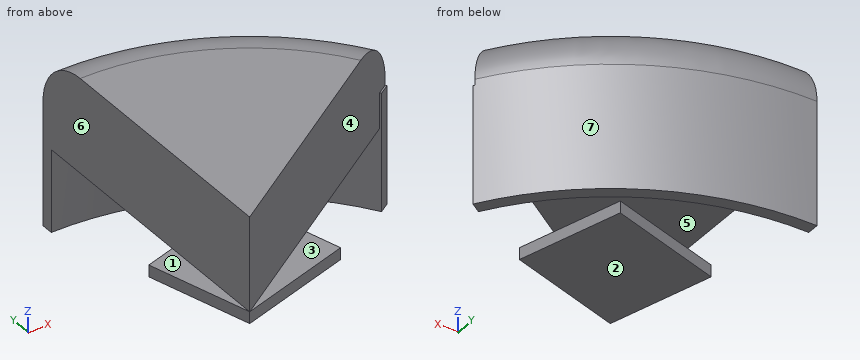
from build123d import *

# Parameters (mm, degrees)
BOX002_W               = 10
BOX002_H               = 9
BOX002_DEPTH           = 1
BOX002_PLACEMENT_ANGLE = 16
CYLINDER001_R          = 22
CYLINDER001_DEPTH      = 37
CYLINDER_R             = 25
CYLINDER_DEPTH         = 40
CYLINDER004_R          = 21
CYLINDER004_DEPTH      = 21
CYLINDER003_R          = 23
CYLINDER003_DEPTH      = 10
CYLINDER002_R          = 25
CYLINDER002_DEPTH      = 5
FILLET_R               = 4.5
BOX001_W               = 37
BOX001_H               = 39
BOX001_DEPTH           = 10
BOX001_PLACEMENT_ANGLE = 57
BOX_W                  = 37
BOX_H                  = 39
BOX_DEPTH              = 10
BOX004_W               = 33
BOX004_H               = 70
BOX004_DEPTH           = 17
BOX003_W               = 33
BOX003_H               = 70
BOX003_DEPTH           = 17
BOX003_PLACEMENT_ANGLE = 57
CYLINDER006_R          = 24
CYLINDER006_DEPTH      = 10
CYLINDER005_R          = 25
CYLINDER005_DEPTH      = 10


with BuildPart() as cubo002:
    # Box002 → Box002 (new body)
    with BuildSketch(Plane.XY):
        with Locations((5, 4.5)):
            Rectangle(BOX002_W, BOX002_H)
    extrude(amount=BOX002_DEPTH)


with BuildPart() as cubo002_1:
    # Box002 placement: moved
    add(cubo002.part.moved(Location((0, 0, 36))).rotate(Axis((0, 0, 36), (0, 0, 1)), BOX002_PLACEMENT_ANGLE))


with BuildPart() as cilindro001:
    # Cylinder001 → Cylinder001 (new body)
    with BuildSketch(Plane.XY):
        Circle(CYLINDER001_R)
    extrude(amount=CYLINDER001_DEPTH)


with BuildPart() as cut:
    # Cylinder → Cylinder (new body)
    with BuildSketch(Plane.XY):
        Circle(CYLINDER_R)
    extrude(amount=CYLINDER_DEPTH)

    # Cut: cut Cilindro001
    add(cilindro001.part, mode=Mode.SUBTRACT)


with BuildPart() as cilindro004:
    # Cylinder004 → Cylinder004 (new body)
    with BuildSketch(Plane.XY):
        Circle(CYLINDER004_R)
    extrude(amount=CYLINDER004_DEPTH)


with BuildPart() as cut001:
    # Cylinder003 → Cylinder003 (new body)
    with BuildSketch(Plane.XY):
        Circle(CYLINDER003_R)
    extrude(amount=CYLINDER003_DEPTH)

    # Cut001: cut Cilindro004
    add(cilindro004.part, mode=Mode.SUBTRACT)


with BuildPart() as cut001_1:
    # Cut001 placement: moved
    add(cut001.part.moved(Location((0, 0, -5))))


with BuildPart() as fusion:
    # Cylinder002 → Cylinder002 (new body)
    with BuildSketch(Plane.XY.offset(40)):
        Circle(CYLINDER002_R)
    extrude(amount=CYLINDER002_DEPTH)

    # Fillet
    fillet_edges = [fusion.edges().sort_by_distance(p)[0] for p in [
        (-25, 0, 45),
    ]]
    fillet(fillet_edges, radius=FILLET_R)

    # Fusion: union Cut, Cut001
    add(cut.part)
    add(cut001_1.part)


with BuildPart() as cubo001:
    # Box001 → Box001 (new body)
    with BuildSketch(Plane.XY):
        with Locations((18.5, 19.5)):
            Rectangle(BOX001_W, BOX001_H)
    extrude(amount=BOX001_DEPTH)


with BuildPart() as cubo001_1:
    # Box001 placement: moved
    add(cubo001.part.moved(Location((0, 0, 37))).rotate(Axis((0, 0, 37), (0, 0, -1)), BOX001_PLACEMENT_ANGLE))


with BuildPart() as common:
    # Box → Box (new body)
    with BuildSketch(Plane.XY.offset(37)):
        with Locations((18.5, 19.5)):
            Rectangle(BOX_W, BOX_H)
    extrude(amount=BOX_DEPTH)

    # Cut002: cut Cubo001
    add(cubo001_1.part, mode=Mode.SUBTRACT)

    # Common: intersect Fusion
    add(fusion.part, mode=Mode.INTERSECT)


with BuildPart() as cubo004:
    # Box004 → Box004 (new body)
    with BuildSketch(Plane(origin=(-33, -19, 29), x_dir=(1, 0, 0), z_dir=(0, 0, 1))):
        with Locations((16.5, 35)):
            Rectangle(BOX004_W, BOX004_H)
    extrude(amount=BOX004_DEPTH)


with BuildPart() as fusion001:
    # Box003 → Box003 (new body)
    with BuildSketch(Plane.XY):
        with Locations((16.5, 35)):
            Rectangle(BOX003_W, BOX003_H)
    extrude(amount=BOX003_DEPTH)


with BuildPart() as fusion001_1:
    # Box003 placement: moved
    add(fusion001.part.moved(Location((-29, -19, 29))).rotate(Axis((-29, -19, 29), (0, 0, -1)), BOX003_PLACEMENT_ANGLE))

    # Fusion001: union Cubo004
    add(cubo004.part)


with BuildPart() as cilindro006:
    # Cylinder006 → Cylinder006 (new body)
    with BuildSketch(Plane.XY.offset(34)):
        Circle(CYLINDER006_R)
    extrude(amount=CYLINDER006_DEPTH)


with BuildPart() as fusion002:
    # Cylinder005 → Cylinder005 (new body)
    with BuildSketch(Plane.XY.offset(34)):
        Circle(CYLINDER005_R)
    extrude(amount=CYLINDER005_DEPTH)

    # Cut003: cut Cilindro006
    add(cilindro006.part, mode=Mode.SUBTRACT)

    # Cut004: cut Fusion001
    add(fusion001_1.part, mode=Mode.SUBTRACT)


with BuildPart() as fusion002_1:
    # Cut004 placement: moved
    add(fusion002.part.moved(Location((0, 0, -4))))

    # Fusion002: union Cubo002, Common
    add(cubo002_1.part)
    add(common.part)


solid = fusion002_1.part
Source: CAD feature listing. Evaluate the final solid. Frame: model axes, mm. Face numbers are marked on the shaded views. A direction names the side the tool comes from. Round coordinates to 2 decimals unless told otherwise and drop trailing zeros. Loops run counter-clockwise (first coordinate to the right, second up) from the corner with the lowest first, then second, coordinate; pieces in that order, holes last. Notation, with made-up numbers: M 23,-28.75 L 57,-28.75 A19 cw 57,-5.75 Z; hole C 52,-27.75 d7. An arc over 180 degrees is marked long. Return JSON: item names as keys, results as strings. Group by question number.
1. Mould query, pull axis Y, two halves, no side actions, for the marked faces 4, 5, 6 and 7. Classes: released by +Y, released by -Y, zero draft, split by the parting line, or undercut.
2. Pin query (flat end, axial travel): pin 1 (0.7 mm diameter, centred on x = 20.5, y = 13.5, fed in from +Z); pin 2 (1 mm diameter, centred on x = 12.5, y = 14, fed in from -Z); pin 3 (8 mm diameter, centred on x = 14, z = 32, fed in from +Y); pin 4 (1.5 mm diameter, centred on y = 7.5, z = 35, fed in from +X). Return the tip coordinate at first contact, or that it passes through.
3. Reachability of the marked faces 1, 2 and 3 from +Z, -Z, +X, -X, +Y, -Y: full face, straight path, thin tool, end or side. Return the list, or none.
4. Section query A-A on y = 4.75. Output: boundary loops of the cut face in (x, z).
5. Material intervals for line 1 along Z through (x, y) = (4.25, 8.5); line 2 along Z through (x, y) = (-0.5, 3); line 3 along X through (y, z) = (14, 34.75), sorted ascending. Write a range as from..to.
6. Section query D-D on z = 41.5. Output: boundary loops of the cut face in (x, y).
7. Section query C-C on z = 38.25. Output: boundary loops of the cut face in (x, y).
8. Section query B-B on z = 35.5. Output: boundary loops of the cut face in (x, y).
Checks:
{
 "1": {"face 4": "released by -Y", "face 5": "undercut", "face 6": "zero draft", "face 7": "released by +Y"},
 "2": {"pin 1": "stops at z = 43.07", "pin 2": "stops at z = 37", "pin 3": "stops at y = 22.91", "pin 4": "passes through"},
 "3": {"face 1": "+Z, -X, +Y, -Y", "face 2": "-Z, +X, -X, -Y", "face 3": "+Z, +X, -Y"},
 "4": {"outline": "M -1.36,36 L 9.04,36 L 9.04,37 L 7.31,37 L 7.31,45 L 0,45 L 0,37 L -1.36,37 Z"},
 "5": {"line 1": "z = 36..45", "line 2": "z = 36..37", "line 3": "x = 19.49..20.71"},
 "6": {"outline": "M 0,0 L 20.87,13.55 A24.89 ccw 0,24.89 Z"},
 "7": {"outline": "M 0,0 L 20.13,13.07 A24 cw 20.2,12.95 L 21.04,13.5 A25 ccw 0,25 Z"},
 "8": {"outline": "M 0,24 A24 cw 20.2,12.95 L 21.04,13.5 A25 ccw 0,25 Z"}
}
